For this review, take the finished solid that the model builds, in its own axes (mm). Give positions to 0.01 mm unless a question says otherwise; leave off trailing zeros. Loops run counter-clockwise (first coordinate to the right, second up) from the corner with the lowest first, then second, coordinate; pieces in that order, holes last. Notation, with made-up numbers: M 48.25,58 L 92.25,58 A24 cw 92.25,86 Z; hole C -23,65 d1. An arc over 180 degrees is marked long. Use CSV: the item, a comma, the result in double quotes. Start each with the question number.
1. Insertion check: P1, Ø6, axis at x = 134, y = 18, coming from the +Z side; P2, Ø3, axis at x = 171, y = -21, coming from the -Z side; P3, Ø3, axis at x = 71.5, y = 12, coming from the +Z side. Each pin has a flat end and moves straight along its axis. Give the tip position at first contact, or say it passes through.
2. Take a section at C-C, the plane x = 184. Write out the cut boundary in (y, z), and give its area (3 significant figures).
3. To check wall thickness, follow line 1 (X direction, y = 6, z = -0.5); line 2 (X direction, y = -31.5, z = 30.5); line 3 (X direction, y = -12, z = 26.5). State the ranges of each line that lie inside material, in increasing order. Write a range as [from, to].
4. Take a section at D-D, the plane z = -36. State how many separate pieces and enclosed holes the cut face has, and give its area (3 significant figures).
5. Take a section at A-A, the plane y = 0. Write out the cut boundary in (x, z).
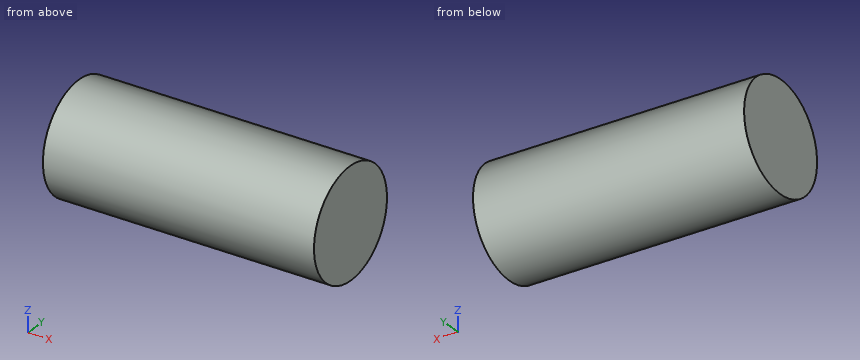
from build123d import *


with BuildPart() as part:
    # ｽｹｯﾁ1 → 回転1 (revolve)
    with BuildSketch(Plane.XY, mode=Mode.PRIVATE) as revolve_1_sk:
        Polygon((10, 0), (0, 0), (0, -60), (150, -60), (150, -10), (140, -10), (100, -50), (10, -50), align=None)
        Polygon((150, -10), (150, -60), (300, -60), (300, 0), (290, 0), (290, -50), (200, -50), (160, -10), align=None)
    revolve(revolve_1_sk.sketch.rotate(Axis((10, 0, 0), (-1, 0, 0)), 180), axis=Axis((10, 0, 0), (-1, 0, 0)))


solid = part.part
Result set:
1,P1,"z = 58.09"
1,P2,"z = -56.74"
1,P3,"z = 59.07"
2,outline,"C 0,0 d120; hole C 0,0 d68"
2,area,"7,680 mm2"
3,line 1,"[0, 10], [290, 300]"
3,line 2,"[0, 10], [106.15, 193.85], [290, 300]"
3,line 3,"[0, 10], [120.91, 179.09], [290, 300]"
4,separate pieces,"1"
4,enclosed holes,"2"
4,area,"15,100 mm2"
5,outline,"M 0,-60 L 300,-60 L 300,60 L 0,60 Z; hole M 10,-50 L 100,-50 L 140,-10 L 160,-10 L 200,-50 L 290,-50 L 290,50 L 200,50 L 160,10 L 140,10 L 100,50 L 10,50 Z"
